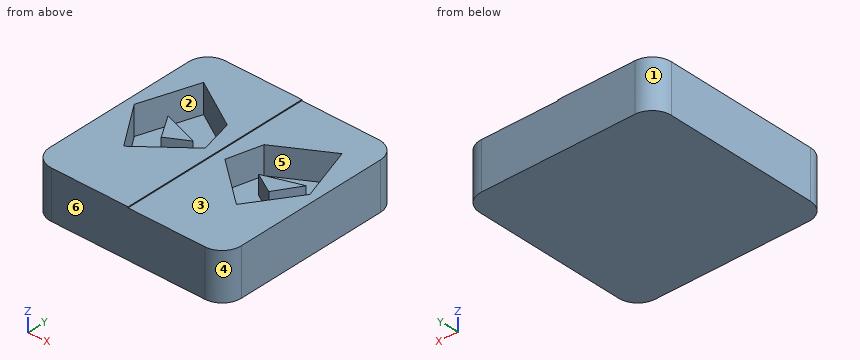
```python
from build123d import *

# Parameters (mm, degrees)
F1_DEPTH = 6.35
F2_DEPTH = 3.81
F3_DEPTH = 1.3208
F4_DEPTH = 0.127


with BuildPart() as f1:
    # F0 (on Top) → F1 (new body)
    with BuildSketch(Plane.XY):
        with BuildLine():
            Line((0, 12.7), (-10.16, 12.7))
            ThreePointArc((-10.16, 12.7), (-11.9560512242, 11.9560512242), (-12.7, 10.16))
            Line((-12.7, 10.16), (-12.7, -10.16))
            ThreePointArc((-12.7, -10.16), (-11.9560512242, -11.9560512242), (-10.16, -12.7))
            Line((-10.16, -12.7), (0, -12.7))
            Line((0, -12.7), (0, 12.7))
        make_face()
        Polygon((-9.1738812898, 8.45533709), (-2.4342421361, 4.4829672283), (-1.3116230257, 0), (-7.4698259894, -5.1080854787), (-11.6343700355, 1.0291366232), align=None, mode=Mode.SUBTRACT)
        with BuildLine():
            Line((10.16, 12.7), (0, 12.7))
            Line((0, 12.7), (0, -12.7))
            Line((0, -12.7), (10.16, -12.7))
            ThreePointArc((10.16, -12.7), (11.9560512242, -11.9560512242), (12.7, -10.16))
            Line((12.7, -10.16), (12.7, 10.16))
            ThreePointArc((12.7, 10.16), (11.9560512242, 11.9560512242), (10.16, 12.7))
        make_face()
        Polygon((7.4698259894, -5.1080854787), (1.3116230257, 0), (2.4342421361, 4.4829672283), (9.1738812898, 8.45533709), (11.6343700355, 1.0291366232), align=None, mode=Mode.SUBTRACT)
        Polygon((-1.3116230257, 0), (-2.4342421361, 4.4829672283), (-9.1738812898, 8.45533709), (-11.6343700355, 1.0291366232), (-7.4698259894, -5.1080854787), align=None)
        Polygon((-4.3419757446, 1.5814950152), (-7.1237651675, 0), (-9.1477709961, 3.227925093), align=None, mode=Mode.SUBTRACT)
        Polygon((-9.1477709961, 3.227925093), (-7.1237651675, 0), (-4.3419757446, 1.5814950152), align=None)
        Polygon((2.4342421361, 4.4829672283), (1.3116230257, 0), (7.4698259894, -5.1080854787), (11.6343700355, 1.0291366232), (9.1738812898, 8.45533709), align=None)
        Polygon((4.3419757446, 1.5814950152), (9.1477709961, 3.227925093), (7.1237651675, 0), align=None, mode=Mode.SUBTRACT)
        Polygon((7.1237651675, 0), (9.1477709961, 3.227925093), (4.3419757446, 1.5814950152), align=None)
    extrude(amount=-F1_DEPTH)

    # F0 (on Top) → F2 (cut)
    with BuildSketch(Plane.XY):
        Polygon((-1.3116230257, 0), (-2.4342421361, 4.4829672283), (-9.1738812898, 8.45533709), (-11.6343700355, 1.0291366232), (-7.4698259894, -5.1080854787), align=None)
        Polygon((-4.3419757446, 1.5814950152), (-7.1237651675, 0), (-9.1477709961, 3.227925093), align=None, mode=Mode.SUBTRACT)
        Polygon((2.4342421361, 4.4829672283), (1.3116230257, 0), (7.4698259894, -5.1080854787), (11.6343700355, 1.0291366232), (9.1738812898, 8.45533709), align=None)
        Polygon((4.3419757446, 1.5814950152), (9.1477709961, 3.227925093), (7.1237651675, 0), align=None, mode=Mode.SUBTRACT)
    extrude(amount=-F2_DEPTH, mode=Mode.SUBTRACT)

    # F0 (on Top) → F3 (cut)
    with BuildSketch(Plane.XY):
        Polygon((-9.1477709961, 3.227925093), (-7.1237651675, 0), (-4.3419757446, 1.5814950152), align=None)
        Polygon((7.1237651675, 0), (9.1477709961, 3.227925093), (4.3419757446, 1.5814950152), align=None)
    extrude(amount=-F3_DEPTH, mode=Mode.SUBTRACT)

    # F0 (on Top) → F4 (cut)
    with BuildSketch(Plane.XY):
        with BuildLine():
            Line((10.16, 12.7), (0, 12.7))
            Line((0, 12.7), (0, -12.7))
            Line((0, -12.7), (10.16, -12.7))
            ThreePointArc((10.16, -12.7), (11.9560512242, -11.9560512242), (12.7, -10.16))
            Line((12.7, -10.16), (12.7, 10.16))
            ThreePointArc((12.7, 10.16), (11.9560512242, 11.9560512242), (10.16, 12.7))
        make_face()
        Polygon((7.4698259894, -5.1080854787), (1.3116230257, 0), (2.4342421361, 4.4829672283), (9.1738812898, 8.45533709), (11.6343700355, 1.0291366232), align=None, mode=Mode.SUBTRACT)
    extrude(amount=-F4_DEPTH, mode=Mode.SUBTRACT)


solid = f1.part
```
The listing builds one solid part. Answer for the finished solid, in the listing's coordinates (mm). Face numbers are marked on the shaded views. A direction names the side the tool comes from. Coordinates: 2 decimals unless noted, no trailing zeros. Write each loop counter-clockwise with the first axis right and the second up, starting at its lowest first coordinate (ties: lowest second). Pieces come first, ordered by that corner, then holes.
Q1. Section C-C, the plane x = 4.75 is taken. Write down the section's boundary in (y, z).
Returned:
outline: (-12.7, -6.35) - (12.7, -6.35) - (12.7, -0.13) - (5.85, -0.13) - (5.85, -3.81) - (1.72, -3.81) - (1.72, -1.32) - (1.35, -1.32) - (1.35, -3.81) - (-2.85, -3.81) - (-2.85, -0.13) - (-12.7, -0.13) - close
Q2. Section A-A, the plane z = -2.5 is taken. Write down the section's boundary in (x, y), then the cut area to 3 significant figures.
Returned:
outline: (-12.7, -10.16) arc R2.54 ccw to (-10.16, -12.7) - (10.16, -12.7) arc R2.54 ccw to (12.7, -10.16) - (12.7, 10.16) arc R2.54 ccw to (10.16, 12.7) - (-10.16, 12.7) arc R2.54 ccw to (-12.7, 10.16) - close; (-9.15, 3.23) - (-7.12, 0) - (-4.34, 1.58) - close; (4.34, 1.58) - (7.12, 0) - (9.15, 3.23) - close; hole (-11.63, 1.03) - (-7.47, -5.11) - (-1.31, 0) - (-2.43, 4.48) - (-9.17, 8.46) - close; hole (1.31, 0) - (7.47, -5.11) - (11.63, 1.03) - (9.17, 8.46) - (2.43, 4.48) - close
area: 488 mm2
Q3. Which of the six approach directions +Z, -Z, +X, -X, +Y, -Y give full straight-line access (tool end or side, diameter ignored) to the marked faces 5 and 6?
Returned:
face 5: +Z
face 6: +Z, -Z, +X, -X, -Y
Q4. The mould has two halves that part along Y. Classify the marked faces 1, 2, 3 and 4: released by +Y, released by -Y, zero draft, split by the parting line, or undercut.
Returned:
face 1: released by +Y
face 2: undercut
face 3: zero draft
face 4: released by -Y
Q5. Given P1, Ø14, axis at x = 8.5, y = -3, coming from the +Z side; P2, Ø3, axis at x = 4, y = 0, coming from the +Z side; P3, Ø1.6, axis at x = 8, y = 1, coming from the +Z side, each flat-ended and moving along its own axis, determine where each tip first touches the part or whether it passes through.
Returned:
P1: stops at z = -0.13
P2: stops at z = -3.81
P3: stops at z = -1.32
Q6. Section B-B, the plane z = -1 is taken. Write down the section's boundary in (x, y).
Returned:
outline: (-12.7, -10.16) arc R2.54 ccw to (-10.16, -12.7) - (10.16, -12.7) arc R2.54 ccw to (12.7, -10.16) - (12.7, 10.16) arc R2.54 ccw to (10.16, 12.7) - (-10.16, 12.7) arc R2.54 ccw to (-12.7, 10.16) - close; hole (-11.63, 1.03) - (-7.47, -5.11) - (-1.31, 0) - (-2.43, 4.48) - (-9.17, 8.46) - close; hole (1.31, 0) - (7.47, -5.11) - (11.63, 1.03) - (9.17, 8.46) - (2.43, 4.48) - close
Q7. Section D-D, the plane y = 6.5 is taken. Write down the section's boundary in (x, z).
Returned:
outline: (-12.7, -6.35) - (12.7, -6.35) - (12.7, -0.13) - (9.82, -0.13) - (9.82, -3.81) - (5.86, -3.81) - (5.86, -0.13) - (0, -0.13) - (0, 0) - (-5.86, 0) - (-5.86, -3.81) - (-9.82, -3.81) - (-9.82, 0) - (-12.7, 0) - close
Q8. Find the intervals of material crossed by line 1 along Y through (x, z) = (8.25, -1.5); line 2 along X through (y, z) = (1.25, -0.5); line 3 along X through (y, z) = (-0.5, -0.5), in increasing order.
Returned:
line 1: y = -12.7 to -3.96, 1.8 to 2.92, 7.91 to 12.7
line 2: x = -12.7 to -11.56, -1.62 to 1.62, 11.56 to 12.7
line 3: x = -12.7 to -10.6, -1.91 to 1.91, 10.6 to 12.7
